Could you check a few things on this model? Use its own coordinates, in mm. A direction names the side the tool comes from. Coordinates: 2 decimals unless noted, no trailing zeros. Loops run counter-clockwise (first coordinate to the right, second up) from the corner with the lowest first, then second, coordinate; pieces in that order, holes last.
1) Imagine slicing it at B-B on y = 19.5. Please give me the cut outline in (x, z), plus the area to 3 significant figures.
2) Will these pins go through, and if not, where does the flat tip stop? P1, Ø3, axis at x = 38, y = 28.5, coming from the +Z side; P2, Ø1.5, axis at x = 28.5, y = 26, coming from the +Z side; P3, Ø6, axis at x = 46.5, z = 7.5, coming from the -Y side; P4, Ø1, axis at y = 29, z = 8, coming from the +X side.
3) Imagine slicing it at A-A on x = 12. Please give me the cut outline in (y, z), plus the area to 3 significant figures.
4) Imagine slicing it at C-C on z = 11. Please give me the cut outline in (x, y), plus the area to 3 significant figures.
5) Thinking about a two-plate mould opening in X: for faces 1 (the face through (43, 25.5, 1)), 2 (the face through (30.533, 9.411, 9.395)), 3 (the face through (29, 18, 0)), 4 (the face through (1, 2, 1)), which applies, released by +X, released by -X, zero draft, split by the parting line, or undercut?
6) If I drill on line 1 along X through (y, z) = (20, 0.75); line 2 along Z through (x, y) = (28, 6.5); line 3 along X through (y, z) = (6, 13.75), over which ranges is the centre line in solid material (lowest first)?
7) Imagine slicing it at D-D on x = 29. Please give me the cut outline in (y, z), plus the area to 3 significant figures.
8) For faces 5 (the face through (15, 9.5, 1)), 6 (the face through (5, 5, 17)), 7 (the face through (29, 18, 2)), which set-ups out of +Z, -Z, +X, -X, +Y, -Y let a thin tool reach every point of the face, with its end or its side?
```python
from build123d import *

# Parameters (mm, degrees)
SKIZZE1_W                        = 58
SKIZZE1_H                        = 35
AUFSATZ_LINEAR_AUSTRAGEN1_DEPTH  = 2
VERRUNDUNG1_R                    = 5
SKIZZE10_R                       = 1.496771876
AUFSATZ_LINEAR_AUSTRAGEN6_DEPTH  = 15
SKIZZE11_R                       = 1.503510887
AUFSATZ_LINEAR_AUSTRAGEN7_DEPTH  = 15
SKIZZE12_R                       = 1.498287051
AUFSATZ_LINEAR_AUSTRAGEN8_DEPTH  = 15
SKIZZE13_R                       = 1.500467236
AUFSATZ_LINEAR_AUSTRAGEN9_DEPTH  = 15
SKIZZE23_W                       = 13
SKIZZE23_H                       = 16
SCHNITT_LINEAR_AUSTRAGEN3_DEPTH  = 15
VERRUNDUNG4_R                    = 1
SKIZZE24_R                       = 1.501958256
AUFSATZ_LINEAR_AUSTRAGEN10_DEPTH = 1
SKIZZE26_R                       = 1.499079917
AUFSATZ_LINEAR_AUSTRAGEN11_DEPTH = 15


with BuildPart() as part:
    # Skizze1 → Aufsatz-Linear austragen1 (new body)
    with BuildSketch(Plane.XY):
        with Locations((29, 17.5)):
            Rectangle(SKIZZE1_W, SKIZZE1_H)
    extrude(amount=AUFSATZ_LINEAR_AUSTRAGEN1_DEPTH)

    # Verrundung1
    verrundung1_edges = [part.edges().sort_by_distance(p)[0] for p in [
        (0, 0, 1),
        (58, 0, 1),
        (58, 35, 1),
        (0, 35, 1),
    ]]
    fillet(verrundung1_edges, radius=VERRUNDUNG1_R)

    # Skizze10 → Aufsatz-Linear austragen6 (add)
    with BuildSketch(Plane.XY.offset(2)):
        with Locations(Location((53, 30, 0), (0, 0, 180))):
            Circle(SKIZZE10_R)
    extrude(amount=AUFSATZ_LINEAR_AUSTRAGEN6_DEPTH)

    # Skizze11 → Aufsatz-Linear austragen7 (add)
    with BuildSketch(Plane.XY.offset(2)):
        with Locations(Location((4.999967007, 30, 0), (0, 0, 180))):
            Circle(SKIZZE11_R)
    extrude(amount=AUFSATZ_LINEAR_AUSTRAGEN7_DEPTH)

    # Skizze12 → Aufsatz-Linear austragen8 (add)
    with BuildSketch(Plane.XY.offset(2)):
        with Locations(Location((5, 5, 0), (0, 0, 180))):
            Circle(SKIZZE12_R)
    extrude(amount=AUFSATZ_LINEAR_AUSTRAGEN8_DEPTH)

    # Skizze13 → Aufsatz-Linear austragen9 (add)
    with BuildSketch(Plane.XY.offset(2)):
        with Locations(Location((53, 5, 0), (0, 0, 180))):
            Circle(SKIZZE13_R)
    extrude(amount=AUFSATZ_LINEAR_AUSTRAGEN9_DEPTH)

    # Skizze23 → Schnitt-Linear austragen3 (cut)
    with BuildSketch(Plane.XY.offset(2)):
        with Locations((42.835818152, 17.5)):
            Rectangle(SKIZZE23_W, SKIZZE23_H)
        with Locations((15.164181848, 17.5)):
            Rectangle(SKIZZE23_W, SKIZZE23_H)
    extrude(amount=-SCHNITT_LINEAR_AUSTRAGEN3_DEPTH, mode=Mode.SUBTRACT)

    # Verrundung4
    verrundung4_edges = [part.edges().sort_by_distance(p)[0] for p in [
        (49.335818152, 25.5, 1),
        (49.335818152, 9.5, 1),
        (36.335818152, 9.5, 1),
        (36.335818152, 25.5, 1),
        (21.664181848, 25.5, 1),
        (21.664181848, 9.5, 1),
        (8.664181848, 9.5, 1),
        (8.664181848, 25.5, 1),
    ]]
    fillet(verrundung4_edges, radius=VERRUNDUNG4_R)

    # Skizze24 → Aufsatz-Linear austragen10 (add)
    with BuildSketch(Plane.XY.offset(2)):
        with Locations(Location((29.015481973, 25.496020028, 0), (0, 0, 180))):
            Circle(SKIZZE24_R)
    extrude(amount=AUFSATZ_LINEAR_AUSTRAGEN10_DEPTH)

    # Skizze26 → Aufsatz-Linear austragen11 (add)
    with BuildSketch(Plane.XY.offset(2)):
        with Locations(Location((29.034976799, 9.476495672, 0), (0, 0, 180))):
            Circle(SKIZZE26_R)
    extrude(amount=AUFSATZ_LINEAR_AUSTRAGEN11_DEPTH)


solid = part.part
```
Filled in:
1. outline: (0, 0) - (8.66, 0) - (8.66, 2) - (0, 2) - close; (21.66, 0) - (36.34, 0) - (36.34, 2) - (21.66, 2) - close; (49.34, 0) - (58, 0) - (58, 2) - (49.34, 2) - close
1. area: 64.0 mm2
2. P1: stops at z = 2
2. P2: stops at z = 3
2. P3: passes through
2. P4: stops at x = 54.41
3. outline: (0, 0) - (9.5, 0) - (9.5, 2) - (0, 2) - close; (25.5, 0) - (35, 0) - (35, 2) - (25.5, 2) - close
3. area: 38.0 mm2
4. outline: circle Ø3 at (5, 5); circle Ø3.01 at (5, 30); circle Ø3 at (29.03, 9.48); circle Ø3 at (53, 5); circle Ø2.99 at (53, 30)
4. area: 35.3 mm2
5. face 1: undercut
5. face 2: split by the parting line
5. face 3: zero draft
5. face 4: released by -X
6. line 1: x = 0 to 8.66, 21.66 to 36.34, 49.34 to 58
6. line 2: z = 0 to 2
6. line 3: x = 3.88 to 6.12, 51.88 to 54.12
7. outline: (0, 0) - (35, 0) - (35, 2) - (27, 2) - (27, 3) - (23.99, 3) - (23.99, 2) - (10.98, 2) - (10.98, 17) - (7.98, 17) - (7.98, 2) - (0, 2) - close
7. area: 118 mm2
8. face 5: +Z, -Z
8. face 6: +Z, +X, -X, +Y, -Y
8. face 7: +Z
